from build123d import *

# Parameters (mm, degrees)
SKETCH1_W           = 85.9
SKETCH1_H           = 26.6
BOSS_EXTRUDE1_DEPTH = 18.4
SHELL1_T            = -2
SKETCH2_R           = 5.75
CUT_EXTRUDE1_DEPTH  = 19.4
CUT_EXTRUDE2_DEPTH  = 86.9
CHAMFER1_SIZE       = 1.5
BOSS_EXTRUDE2_DEPTH = 18.4
SKETCH5_R           = 1.65
CUT_EXTRUDE3_DEPTH  = 19.4
SKETCH6_R           = 2.85
CUT_EXTRUDE4_DEPTH  = 2
CHAMFER2_SIZE       = 0.3
CHAMFER3_SIZE       = 1
SKETCH7_W           = 79.6
SKETCH7_H           = 6.85
CUT_EXTRUDE5_DEPTH  = 4
CHAMFER4_SIZE       = 0.3
SKETCH8_W           = 7.7
SKETCH8_H           = 4
CUT_EXTRUDE6_DEPTH  = 34.45


with BuildPart() as part:
    # Sketch1 → Boss-Extrude1 (new body)
    with BuildSketch(Plane(origin=(0, 0, 0), x_dir=(1, 0, 0), z_dir=(0, 1, 0))):
        with Locations((42.95, 13.3)):
            Rectangle(SKETCH1_W, SKETCH1_H)
    extrude(amount=BOSS_EXTRUDE1_DEPTH)

    # Shell1
    shell1_openings = [part.faces().sort_by_distance(p)[0] for p in [
        (42.95, 0, -13.3),
    ]]
    offset(amount=SHELL1_T, openings=shell1_openings, kind=Kind.INTERSECTION)

    # Sketch2 → Cut-Extrude1 (cut, through all)
    with BuildSketch(Plane(origin=(0, 18.4, 0), x_dir=(1, 0, 0), z_dir=(0, 1, 0))):
        with Locations((42.95, 13.3)):
            Circle(SKETCH2_R)
    extrude(amount=-CUT_EXTRUDE1_DEPTH, mode=Mode.SUBTRACT)

    # Sketch3 → Cut-Extrude2 (cut, through all)
    with BuildSketch(Plane(origin=(85.9, 0, 0), x_dir=(0, 0, -1), z_dir=(1, 0, 0))):
        Polygon((2.8125, 0), (24.6, 8.087162678), (24.6, 0), align=None)
    extrude(amount=-CUT_EXTRUDE2_DEPTH, mode=Mode.SUBTRACT)

    # Chamfer1
    chamfer1_edges = [part.edges().sort_by_distance(p)[0] for p in [
        (37.2, 18.4, -13.3),
    ]]
    chamfer(chamfer1_edges, length=CHAMFER1_SIZE)

    # Sketch4 → Boss-Extrude2 (add)
    with BuildSketch(Plane(origin=(0, 18.4, 0), x_dir=(1, 0, 0), z_dir=(0, 1, 0))):
        with BuildLine():
            Line((3.15, 29.6), (3.15, 26.6))
            Line((3.15, 26.6), (10.85, 26.6))
            Line((10.85, 26.6), (10.85, 29.6))
            ThreePointArc((10.85, 29.6), (7, 33.45), (3.15, 29.6))
        make_face()
        with BuildLine():
            Line((3.15, -3), (3.15, 0))
            Line((3.15, 0), (10.85, 0))
            Line((10.85, 0), (10.85, -3))
            ThreePointArc((10.85, -3), (7, -6.85), (3.15, -3))
        make_face()
        with BuildLine():
            Line((75.05, 0), (75.05, -3))
            ThreePointArc((75.05, -3), (78.9, -6.85), (82.75, -3))
            Line((82.75, -3), (82.75, 0))
            Line((82.75, 0), (75.05, 0))
        make_face()
        with BuildLine():
            Line((75.05, 26.6), (75.05, 29.6))
            ThreePointArc((75.05, 29.6), (78.9, 33.45), (82.75, 29.6))
            Line((82.75, 29.6), (82.75, 26.6))
            Line((82.75, 26.6), (75.05, 26.6))
        make_face()
    extrude(amount=-BOSS_EXTRUDE2_DEPTH)

    # Sketch5 → Cut-Extrude3 (cut, through all)
    with BuildSketch(Plane(origin=(0, 18.4, 0), x_dir=(1, 0, 0), z_dir=(0, 1, 0))):
        with Locations((7, 29.6)):
            Circle(SKETCH5_R)
        with Locations((7, -3)):
            Circle(SKETCH5_R)
        with Locations((78.9, -3)):
            Circle(SKETCH5_R)
        with Locations((78.9, 29.6)):
            Circle(SKETCH5_R)
    extrude(amount=-CUT_EXTRUDE3_DEPTH, mode=Mode.SUBTRACT)

    # Sketch6 → Cut-Extrude4 (cut)
    with BuildSketch(Plane(origin=(0, 18.4, 0), x_dir=(1, 0, 0), z_dir=(0, 1, 0))):
        with Locations((7, 29.6)):
            Circle(SKETCH6_R)
        with Locations((78.9, 29.6)):
            Circle(SKETCH6_R)
        with Locations((78.9, -3)):
            Circle(SKETCH6_R)
        with Locations((7, -3)):
            Circle(SKETCH6_R)
    extrude(amount=-CUT_EXTRUDE4_DEPTH, mode=Mode.SUBTRACT)

    # Chamfer2
    chamfer2_edges = [part.edges().sort_by_distance(p)[0] for p in [
        (4.15, 18.4, 3),
        (76.05, 18.4, 3),
        (76.05, 18.4, -29.6),
        (4.15, 18.4, -29.6),
    ]]
    chamfer(chamfer2_edges, length=CHAMFER2_SIZE)

    # Chamfer3
    chamfer3_edges = [part.edges().sort_by_distance(p)[0] for p in [
        (85.9, 18.4, -13.3),
        (84.325, 18.4, -26.6),
        (0, 18.4, -13.3),
        (1.575, 18.4, -26.6),
        (42.95, 18.4, 0),
        (1.575, 18.4, 0),
        (0, 9.2, -26.6),
        (85.9, 9.2, -26.6),
        (85.9, 9.2, 0),
        (0, 9.2, 0),
        (84.325, 18.4, 0),
        (42.95, 18.4, -26.6),
    ]]
    chamfer(chamfer3_edges, length=CHAMFER3_SIZE)

    # Sketch7 → Cut-Extrude5 (cut)
    with BuildSketch(Plane.XZ):
        with Locations((42.95, 3.425)):
            Rectangle(SKETCH7_W, SKETCH7_H)
        with Locations((42.95, -30.025)):
            Rectangle(SKETCH7_W, SKETCH7_H)
    extrude(amount=-CUT_EXTRUDE5_DEPTH, mode=Mode.SUBTRACT)

    # Chamfer4
    chamfer4_edges = [part.edges().sort_by_distance(p)[0] for p in [
        (7, 18.4, -33.45),
        (3.15, 18.4, -27.6),
        (10.85, 18.4, -27.6),
        (7, 18.4, 6.85),
        (10.85, 18.4, 1),
        (3.15, 18.4, 1),
        (78.9, 18.4, 6.85),
        (82.75, 18.4, 1),
        (75.05, 18.4, 1),
        (78.9, 18.4, -33.45),
        (75.05, 18.4, -27.6),
        (82.75, 18.4, -27.6),
    ]]
    chamfer(chamfer4_edges, length=CHAMFER4_SIZE)

    # Sketch8 → Cut-Extrude6 (cut, through all)
    with BuildSketch(Plane.XY):
        with Locations((7, 2)):
            Rectangle(SKETCH8_W, SKETCH8_H)
        with Locations((78.9, 2)):
            Rectangle(SKETCH8_W, SKETCH8_H)
    extrude(amount=-CUT_EXTRUDE6_DEPTH, mode=Mode.SUBTRACT)


solid = part.part
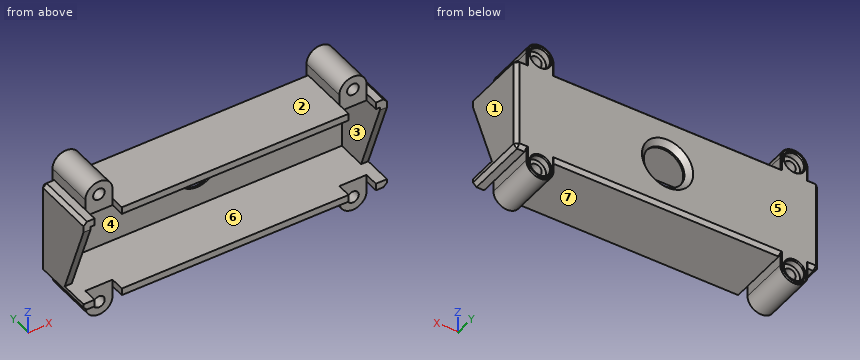
Can you work these out from the model? Positions are in its coordinate system, mm. Face numbers are marked on the shaded views. A direction names the side the tool comes from. Coordinates: 2 decimals unless noted, no trailing zeros. Loops run counter-clockwise (first coordinate to the right, second up) from the corner with the lowest first, then second, coordinate; pieces in that order, holes last. Notation, with made-up numbers: M 65,89 L 104,89 A19 cw 104,96 Z; hole C 44.5,66 d1. An arc over 180 degrees is marked long. Answer as CSV lines item,"result". Start each with the question number.
1. For the marked faces 1, 2 and 3, which set-ups out of +Z, -Z, +X, -X, +Y, -Y let a thin tool reach every point of the face, with its end or its side?
2. Thinking about a two-plate mould opening in Z: for the marked faces 4, 5, 6 and 7, which applies, +Z half, -Z half, draft (parallel to the pull), parting line (faces both ways), or undercut?
3. Suppose I cut it at B-B, the plane x = 42.95. List the corners of the cut face in (y, z) for me, plus the area to 4 significant figures.
4. For pin 1 Ø3 at (x, y) = (42.5, 3) entering from -Z; pin 2 Ø3 at (y, z) = (10.5, 1) entering from -X; pin 3 Ø1.1 at (y, z) = (10, -27.5) entering from +X, each with a flat end and sliding along its axis, tell me the tip position at first contact or that it passes through.
5. Suppose I cut it at D-D, the plane z = -13.3. List the corners of the cut face in (x, y) for me, plus the area to 3 significant figures.
6. Suppose I cut it at A-A, the plane x = 7. Count the separate pieces of the cut face and the enclosed holes in it, plus the area to 3 significant figures.
7. If I drill on probe 1 along Z at (x, y) = (7, 17.7); probe 2 along X at (y, z) = (17.25, 3); probe 3 along Z at (x, y) = (7, 9.75), over which ranges is the centre line in solid material (lowest first)? Write a range as [from, to].
Output:
1,face 1,"+Z, -Z, +X, +Y, -Y"
1,face 2,"+Z, +Y, -Y"
1,face 3,"-Y"
2,face 4,"undercut"
2,face 5,"draft"
2,face 6,"undercut"
2,face 7,"-Z half"
3,outline,"M 0,-26.6 L 17.4,-26.6 L 18.4,-25.6 L 18.4,-20.55 L 16.9,-19.05 L 16.4,-19.05 L 16.4,-24.6 L 0,-24.6 Z; M 0,-2 L 16.4,-2 L 16.4,-7.55 L 16.9,-7.55 L 18.4,-6.05 L 18.4,-1 L 17.4,0 L 0,0 Z"
3,area,"92.55 mm^2"
4,pin 1,"stops at z = -26.6"
4,pin 2,"stops at x = 0.5"
4,pin 3,"stops at x = 82.75"
5,outline,"M 0,3.89 L 2,3.89 L 2,16.4 L 37.2,16.4 L 37.2,16.9 L 35.7,18.4 L 1,18.4 L 0,17.4 Z; M 48.7,16.4 L 83.9,16.4 L 83.9,3.89 L 85.9,3.89 L 85.9,17.4 L 84.9,18.4 L 50.2,18.4 L 48.7,16.9 Z"
5,area,"196 mm^2"
6,separate pieces,"3"
6,enclosed holes,"0"
6,area,"195 mm^2"
7,probe 1,"z = [-33.45, -32.45], [-26.75, 0.15], [5.85, 6.85]"
7,probe 2,"x = [3.15, 4.15], [9.85, 10.85], [75.05, 76.05], [81.75, 82.75]"
7,probe 3,"z = [-33.45, -31.25], [-27.95, -24.6], [-2, 1.35], [4.65, 6.85]"
